```python
from build123d import *

# Parameters (mm, degrees)
SKETCH1_W           = 30
SKETCH1_H           = 8
BOSS_EXTRUDE1_DEPTH = 2
SKETCH2_R           = 1.5
CUT_EXTRUDE1_DEPTH  = 32.112698372
SKETCH3_R           = 1
CUT_EXTRUDE2_DEPTH  = 32.112698372
FILLET1_R           = 2


with BuildPart() as part:
    # Sketch1 → Boss-Extrude1 (new body)
    with BuildSketch(Plane(origin=(0, 0, 0), x_dir=(1, 0, 0), z_dir=(0, 1, 0))):
        with Locations((15, -4)):
            Rectangle(SKETCH1_W, SKETCH1_H)
    extrude(amount=BOSS_EXTRUDE1_DEPTH)

    # Sketch2 → Cut-Extrude1 (cut, through all)
    with BuildSketch(Plane(origin=(0, 2, 0), x_dir=(1, 0, 0), z_dir=(0, 1, 0))):
        with Locations(Location((25, -4, 0), (0, 0, 270))):
            Circle(SKETCH2_R)
    extrude(amount=-CUT_EXTRUDE1_DEPTH, mode=Mode.SUBTRACT)

    # Sketch3 → Cut-Extrude2 (cut, through all)
    with BuildSketch(Plane(origin=(0, 2, 0), x_dir=(1, 0, 0), z_dir=(0, 1, 0))):
        with Locations(Location((5, -4, 0), (0, 0, 270))):
            Circle(SKETCH3_R)
    extrude(amount=-CUT_EXTRUDE2_DEPTH, mode=Mode.SUBTRACT)

    # Fillet1
    fillet1_edges = [part.edges().sort_by_distance(p)[0] for p in [
        (0, 1, 0),
        (30, 1, 0),
        (30, 1, 8),
        (0, 1, 8),
    ]]
    fillet(fillet1_edges, radius=FILLET1_R)


solid = part.part
```
Geometry check sheet. Reference: the model listing, model coordinates, mm. Coordinates: 2 decimals unless noted, no trailing zeros. Order: outer loops, then holes, each group sorted by start corner. A loop starts at its lowest first (then second) coordinate and runs counter-clockwise, first axis right, second up. Notation, with made-up numbers: (5, 58.25) - (51, 58.25) arc R36 cw to (51, 97.25) - close; hole circle Ø2 at (38, -27). An arc over 180 degrees is marked (long way). Use one line per item in the form item = value.
1. Section check A-A (x = 5). Record the boundary of the cut face in (y, z), then the cut area to 3 significant figures.
Here are the results:
outline = (0, 0) - (2, 0) - (2, 3) - (0, 3) - close; (0, 5) - (2, 5) - (2, 8) - (0, 8) - close
area = 12.0 mm²
2. Section check B-B (z = 4). Record the boundary of the cut face in (x, y), then the cut area to 3 significant figures.
Here are the results:
outline = (0, 0) - (4, 0) - (4, 2) - (0, 2) - close; (6, 0) - (23.5, 0) - (23.5, 2) - (6, 2) - close; (26.5, 0) - (30, 0) - (30, 2) - (26.5, 2) - close
area = 50.0 mm²
3. Scan lines: line 1 (X direction, y = 1.45, z = 4); line 2 (X direction, y = 0.3, z = 5.25); line 3 (X direction, y = 1.4, z = 1.75). Record each from-to range of solid material in increasing order.
Here are the results:
line_1 = 0 to 4, 6 to 23.5, 26.5 to 30
line_2 = 0 to 24.17, 25.83 to 30
line_3 = 0.02 to 29.98
4. Section check D-D (z = 5.25). Record the boundary of the cut face in (x, y), then the cut area to 3 significant figures.
Here are the results:
outline = (0, 0) - (24.17, 0) - (24.17, 2) - (0, 2) - close; (25.83, 0) - (30, 0) - (30, 2) - (25.83, 2) - close
area = 56.7 mm²
5. Draft check along Z on faces 1 (the face through (29.4, 1.01, 0.57)), 2 (the face through (5.676, 1.014, 3.263)), 3 (the face through (0.57, 1.01, 7.4)), 4 (the face through (30, 1, 4)). Enter one of: pulls with the +Z half, pulls with the -Z half, needs draft (parallel to the pull), parting line crosses it, or undercut.
Here are the results:
face_1 = pulls with the -Z half
face_2 = undercut
face_3 = pulls with the +Z half
face_4 = needs draft
6. Section check C-C (y = 1.1). Record the boundary of the cut face in (x, z).
Here are the results:
outline = (0, 2) arc R2 ccw to (2, 0) - (28, 0) arc R2 ccw to (30, 2) - (30, 6) arc R2 ccw to (28, 8) - (2, 8) arc R2 ccw to (0, 6) - close; hole circle Ø2 at (5, 4); hole circle Ø3 at (25, 4)
